Autodesk Inventor part; units mm, degrees
ref_plane "Work Plane1" through (0, 0, 0) normal (0, 0, 1) x (1, 0, 0)
ref_plane "YZ Plane" through (0, 0, 0) normal (1, 0, 0) x (0, 1, 0)
ref_plane "XZ Plane" through (0, 0, 0) normal (0, 1, 0) x (-1, 0, 0)
ref_plane "Work Plane1" through (0, 0, 0) normal (0, 0, 1) x (1, 0, 0)
sketch "Sketch1" plane through (0, 0, 0) normal (0, 0, 1) x (1, 0, 0)
  circle A0 centre (228.1, 21.9203) radius 2.3114
  circle A1 centre (431.3, 21.9203) radius 2.3114
  line L0 (318.0242, 34.6203) -> (379.4758, 34.6203)
  line L1 (215.4, 19.6089) -> (215.4, 11.6079)
  line L2 (444, 9.2203) -> (444, 11.6079)
  line L3 (221.75, 34.6203) -> (437.65, 34.6203)
  line L4 (444, 28.2703) -> (444, -35.2297)
  line L5 (437.65, -41.5797) -> (255.2197, -41.5797)
  line L6 (215.4, 3.0597) -> (215.4, 28.2703)
  line L7 (190.0994, 1.6338) -> (231.0454, -48.1215) construction
  arc A2 (437.65, -41.5797) -> (444, -35.2297) centre (437.65, -35.2297) ccw
  arc A3 (221.75, 34.6203) -> (215.4, 28.2703) centre (221.75, 28.2703) ccw
  arc A4 (444, 28.2703) -> (437.65, 34.6203) centre (437.65, 28.2703) ccw
  line L8 (218.8779, -3.3569) -> (250.4419, -39.4124)
  line L9 (218.8779, -3.3569) -> (216.9197, -1.0623)
  arc A5 (250.4419, -39.4124) -> (255.2197, -41.5797) centre (255.2197, -35.2297) ccw
  arc A6 (215.4, 3.0597) -> (216.9197, -1.0623) centre (221.75, 3.0597) ccw
  point P0 (0, 0)
  point P1 (444, -41.5797)
  point P2 (444, 34.6203)
  point P3 (444, 10.4141)
  point P4 (215.4, 15.6084)
  point P5 (379.4758, 34.6203)
  point P6 (252.3392, -41.5797)
  dimension "d0" = 76.2
  dimension "d1" = 0
  dimension "d3" = 0
  dimension "d5" = 6.35
  dimension "d6" = 6.35
  dimension "d19" = 50.8
  dimension "d21" = 6.35
extrude "Plate1" add sketch "Sketch1" along normal blind 1.5875
sketch "Sketch5" plane through (221.75, 34.6203, 1.5875) normal (0, 0, 1) x (1, 0, 0)
  circle A0 centre (6.35, -12.7) radius 2.3114
  circle A1 centre (12.7, -6.35) radius 2.3368
  circle A2 centre (19.05, -12.7) radius 1.5652 construction
  point P0 (-221.75, -34.6203)
  dimension "d22" = 4.6736
  dimension "d31" = 12.7
  dimension "d32" = 6.35
  dimension "d33" = -6.35
sheet face with bend "Face2" sketch "Sketch5" thickness 1.5875 toward (0, 0, -1) bend radius 1.5875 contours A0
bend "Bend1"
extrude "Cut1" cut sketch "Sketch5" against normal blind 1.5875 contours A1
sketch "Sketch6" plane through (0, 0, 1.5875) normal (0, 0, 1) x (1, 0, 0)
  circle A0 centre (424.95, 28.2703) radius 2.3368
  circle A1 centre (418.6, 21.9203) radius 1.1969 construction
  circle A2 centre (431.3, 21.9203) radius 2.3114
  point P0 (0, 0)
  dimension "d34" = 4.6736
  dimension "d35" = 6.35
  dimension "d36" = 0
  dimension "d37" = 12.7
  dimension "d38" = 6.35
sheet face with bend "Face3" sketch "Sketch6" thickness 1.5875 toward (0, 0, -1) bend radius 1.5875 contours A2
bend "Bend2"
extrude "Cut2" cut sketch "Sketch6" against normal blind 1.5875 contours A0
equation "\"d29\" = Thickness"
equation "\"d44\" = Thickness"
equation "\"d7\" = Thickness"
equation "\"d24\" = BendRadius"
equation "\"d25\" = BendReliefWidth"
equation "\"d27\" = MinimumRemnant"
equation "\"d26\" = BendReliefDepth"
equation "\"d28\" = TransitionRadius"
equation "\"d39\" = BendRadius"
equation "\"d40\" = BendReliefWidth"
equation "\"d42\" = MinimumRemnant"
equation "\"d41\" = BendReliefDepth"
equation "\"d43\" = TransitionRadius"
equation "\"BendRadius\" = Thickness"
equation "\"BendReliefWidth\" = Thickness"
equation "\"BendReliefDepth\" = 0.5 * Thickness"
equation "\"CornerReliefSize\" = 4 * Thickness"
equation "\"MinimumRemnant\" = 2 * Thickness"
equation "\"TransitionRadius\" = BendRadius"
equation "\"JacobiRadiusSize\" = BendRadius"
equation "\"GapSize\" = Thickness"
properties part number "wingpoly"
Here's how the part is built. I have some questions about the finished solid (model axes, mm). Coordinates: 2 decimals unless noted, no trailing zeros. Loops run counter-clockwise (first coordinate to the right, second up) from the corner with the lowest first, then second, coordinate; pieces in that order, holes last. Notation, with made-up numbers: (3.5, 13.25) - (54.5, 13.25) arc R12 ccw to (54.5, 33.25) - close; hole circle Ø5 at (65.5, 68.5). An arc over 180 degrees is marked (long way). Return JSON: item names as keys, results as strings. Group by question number.
Item 1: If we section it at B-B on x = 424.95: Write out the boundary of the cut face in (y, z).
Item 2: If we section it at C-C on x = 234.45: Write out the boundary of the cut face in (y, z).
Item 3: I need wall thicknesses on line 1 (Y direction, x = 424.95, z = 1.1); line 2 (Y direction, x = 234.45, z = 0.9); line 3 (X direction, y = -14, z = 1.1). Which ranges of each line are inside material? Lowest first, please. Write a range as from..to.
Item 4: If we section it at D-D on y = -11: Write out the boundary of the cut face in (x, z).
Item 5: We'd pull the mould along X, two halves only. Please class faces 1 (the face through (328, -3, 1.588)), 2 (the face through (442.19, -39.67, 0.78)), 3 (the face through (232.115, 28.373, 0.805)), 4 (the face through (217.2, 32.7, 0.8)): +X half, -X half, draft (parallel to the pull), parting line (faces both ways), or undercut.
Item 6: If we section it at A-A on z = 1.1: Write out the boundary of the cut face in (x, y), and give its area (3 significant figures).
Calculated:
{
 "1": {"outline": "(-41.58, 0) - (25.93, 0) - (25.93, 1.59) - (-41.58, 1.59) - close; (30.61, 0) - (34.62, 0) - (34.62, 1.59) - (30.61, 1.59) - close"},
 "2": {"outline": "(-21.14, 0) - (25.93, 0) - (25.93, 1.59) - (-21.14, 1.59) - close; (30.61, 0) - (34.62, 0) - (34.62, 1.59) - (30.61, 1.59) - close"},
 "3": {"line 1": "y = -41.58..25.93, 30.61..34.62", "line 2": "y = -21.14..25.93, 30.61..34.62", "line 3": "x = 228.2..444"},
 "4": {"outline": "(225.57, 0) - (444, 0) - (444, 1.59) - (225.57, 1.59) - close"},
 "5": {"face 1": "draft", "face 2": "+X half", "face 3": "undercut", "face 4": "-X half"},
 "6": {"outline": "(215.4, 3.06) arc R6.35 ccw to (216.92, -1.06) - (218.88, -3.36) - (250.44, -39.41) arc R6.35 ccw to (255.22, -41.58) - (437.65, -41.58) arc R6.35 ccw to (444, -35.23) - (444, 28.27) arc R6.35 ccw to (437.65, 34.62) - (221.75, 34.62) arc R6.35 ccw to (215.4, 28.27) - close; hole circle Ø4.67 at (234.45, 28.27); hole circle Ø4.67 at (424.95, 28.27)", "area": "16,600 mm^2"}
}
